Read the model definition and answer for the solid it produces. Units are mm, in the model's axes. A direction names the side the tool comes from. Coordinates: 2 decimals unless noted, no trailing zeros. Order: outer loops, then holes, each group sorted by start corner. A loop starts at its lowest first (then second) coordinate and runs counter-clockwise, first axis right, second up. Notation, with made-up numbers: M 42.5,58 L 72.5,58 A27 cw 72.5,92 Z; hole C 32.5,80 d2. An arc over 180 degrees is marked long. Use a Markdown table: item, result. Add a question column.
1) Each of these flat-tipped pins is pushed along its axis until it touches: pin 1 Ø2 at (x, z) = (0.5, -11) entering from +Y; pin 2 Ø3 at (x, y) = (-9, 5) entering from -Z; pin 3 Ø1.5 at (x, z) = (1, -36) entering from +Y. Where does it stop, or does it pass through?
2) Find the intervals of material crossed by probe 1 along Y at (x, z) = (0, -38.5); probe 2 along X at (y, z) = (2.5, -31); probe 3 along Y at (x, z) = (4, 19.5), in increasing order. Write a range as [from, to].
3) For faces 1 (the face through (0, 3, -25.5)), 2 (the face through (-2.5, 3, -38)), 3 (the face through (2.5, 3, -38)), 4 (the face through (0, 1.7, -1)), determine the directions among +Z, -Z, +X, -X, +Y, -Y from which every point of the face is accessible in a straight line to the end or side of a thin tool.
4) Find section B-B on z = 22. Write down the section's boundary in (x, y), plus the area to 3 significant figures.
5) Find section A-A on z = -15. Write down the section's boundary in (x, y), plus the area to 3 significant figures.
from build123d import *

# Parameters (mm, degrees)
SKETCH1_W           = 30
SKETCH1_H           = 100
BOSS_EXTRUDE1_DEPTH = 1.7
FILLET2_R           = 12
FILLET3_R           = 2
BOSS_EXTRUDE2_DEPTH = 2
SKETCH4_R           = 3.4
BOSS_EXTRUDE3_DEPTH = 6
FILLET4_R           = 1.5


with BuildPart() as part:
    # Sketch1 → Boss-Extrude1 (new body)
    with BuildSketch(Plane(origin=(0, 0, 0), x_dir=(1, 0, 0), z_dir=(0, 1, 0))):
        Rectangle(SKETCH1_W, SKETCH1_H)
    extrude(amount=BOSS_EXTRUDE1_DEPTH)

    # Fillet2
    fillet2_edges = [part.edges().sort_by_distance(p)[0] for p in [
        (-15, 0.85, 50),
        (15, 0.85, 50),
    ]]
    fillet(fillet2_edges, radius=FILLET2_R)

    # Fillet3
    # the kernel refuses this fillet: 2 mm, written as the material it takes off along each edge
    with BuildSketch(Plane(origin=(19.943429983, 0, -50), x_dir=(0, 0, 1), z_dir=(-1, 0, 0))) as fillet3_piece_1:
        with BuildLine():
            CenterArc((1.977371993, 2), FILLET3_R, 188.626926559, 81.373073441)
            Line((0, 1.7), (-0.03954744, 1.694))
            ThreePointArc((-0.03954744, 1.694), (-0.04, 0.85), (-0.04, 0))
            Line((-0.04, 0), (0, -0.04))
            Line((0, -0.04), (1.977371993, -0.04))
            Line((1.977371993, -0.04), (1.977371993, 0))
        make_face()
    extrude(amount=39.886859967, mode=Mode.SUBTRACT)
    with BuildSketch(Plane(origin=(-15, 0, -54.943429983), x_dir=(1, 0, 0), z_dir=(0, 0, 1)), Plane(origin=(15, 0, 38), x_dir=(-1, 0, 0), z_dir=(0, 0, -1))) as fillet3_piece_2:
        with BuildLine():
            CenterArc((1.977371993, 2), FILLET3_R, 188.626926559, 81.373073441)
            Line((0, 1.7), (-0.03954744, 1.694))
            ThreePointArc((-0.03954744, 1.694), (-0.04, 0.85), (-0.04, 0))
            Line((-0.04, 0), (0, -0.04))
            Line((0, -0.04), (1.977371993, -0.04))
            Line((1.977371993, -0.04), (1.977371993, 0))
        make_face()
    extrude(amount=92.943429983, mode=Mode.SUBTRACT)
    with BuildSketch(Plane(origin=(-3, 0, 38), x_dir=(0, 0, 1), z_dir=(1, 0, 0))) as fillet3_piece_3:
        with BuildLine():
            CenterArc((10.022628007, -2), FILLET3_R, 8.626926559, 81.373073441)
            Line((12, -1.7), (12.03954744, -1.694))
            ThreePointArc((12.03954744, -1.694), (12.04, -0.85), (12.04, 0))
            Line((12.04, 0), (12, 0.04))
            Line((12, 0.04), (10.022628007, 0.04))
            Line((10.022628007, 0.04), (10.022628007, 0))
        make_face()
    revolve(axis=Axis((-3, 0, 38), (0, -1, 0)), revolution_arc=90, mode=Mode.SUBTRACT)
    with BuildSketch(Plane(origin=(-3, 0, 50), x_dir=(0, 1, 0), z_dir=(1, 0, 0))) as fillet3_piece_4:
        with BuildLine():
            CenterArc((2, -1.977371993), FILLET3_R, 98.626926559, 81.373073441)
            Line((0, -1.977371993), (-0.04, -1.977371993))
            Line((-0.04, -1.977371993), (-0.04, 0))
            Line((-0.04, 0), (0, 0.04))
            ThreePointArc((0, 0.04), (0.85, 0.04), (1.694, 0.03954744))
            Line((1.694, 0.03954744), (1.7, 0))
        make_face()
    extrude(amount=6, mode=Mode.SUBTRACT)
    with BuildSketch(Plane(origin=(3, 0, 38), x_dir=(0, 0, 1), z_dir=(-1, 0, 0))) as fillet3_piece_5:
        with BuildLine():
            CenterArc((10.022628007, 2), FILLET3_R, 270, 81.373073441)
            Line((12, 1.7), (12.03954744, 1.694))
            ThreePointArc((12.03954744, 1.694), (12.04, 0.85), (12.04, 0))
            Line((12.04, 0), (12, -0.04))
            Line((12, -0.04), (10.022628007, -0.04))
            Line((10.022628007, -0.04), (10.022628007, 0))
        make_face()
    revolve(axis=Axis((3, 0, 38), (0, 1, 0)), revolution_arc=90, mode=Mode.SUBTRACT)

    # Sketch3 → Boss-Extrude2 (add)
    with BuildSketch(Plane(origin=(0, 1.7, 0), x_dir=(1, 0, 0), z_dir=(0, 1, 0))):
        Polygon((-2.5, 50), (2.5, 50), (2.5, 49.5), (2.5, 25.5), (-2.5, 25.5), (-2.5, 49.5), align=None)
    extrude(amount=BOSS_EXTRUDE2_DEPTH)

    # Sketch4 → Boss-Extrude3 (add)
    with BuildSketch(Plane(origin=(0, 1.7, 0), x_dir=(1, 0, 0), z_dir=(0, 1, 0))):
        with Locations(Location((-8.75, 15, 0), (0, 0, 270))):
            Circle(SKETCH4_R)
        with Locations(Location((8.75, 15, 0), (0, 0, 90))):
            Circle(SKETCH4_R)
    extrude(amount=BOSS_EXTRUDE3_DEPTH)

    # Fillet4
    fillet4_edges = [part.edges().sort_by_distance(p)[0] for p in [
        (-8.75, 7.7, -18.4),
        (8.75, 7.7, -11.6),
    ]]
    fillet(fillet4_edges, radius=FILLET4_R)


solid = part.part
Check result:
| question | item | result |
|---|---|---|
| 1 | pin 1 | stops at y = 1.7 |
| 1 | pin 2 | stops at z = -18.4 |
| 1 | pin 3 | stops at y = 3.7 |
| 2 | probe 1 | y = [0, 3.7] |
| 2 | probe 2 | x = [-2.5, 2.5] |
| 2 | probe 3 | y = [0, 1.7] |
| 3 | face 1 | +Z, +X, -X, +Y |
| 3 | face 2 | +Z, -Z, -X, +Y |
| 3 | face 3 | +Z, -Z, +X, +Y |
| 3 | face 4 | +Y |
| 4 | outline | M -15,1.7 A2 ccw -13.02,0 L 13.02,0 A2 ccw 15,1.7 Z |
| 4 | area | 49.4 mm2 |
| 5 | outline | M -15,1.7 A2 ccw -13.02,0 L 13.02,0 A2 ccw 15,1.7 L 12.15,1.7 L 12.15,6.2 A1.5 ccw 10.65,7.7 L 6.85,7.7 A1.5 ccw 5.35,6.2 L 5.35,1.7 L -5.35,1.7 L -5.35,6.2 A1.5 ccw -6.85,7.7 L -10.65,7.7 A1.5 ccw -12.15,6.2 L -12.15,1.7 Z |
| 5 | area | 129 mm2 |
